Source: three-view drawing plus pictorial views. Frame: mm from the lowest corner of the part. A direction names the side the tool comes from. Round coordinates to 2 decimals unless told otherwise and drop trailing zeros. Loops run counter-clockwise (first coordinate to the right, second up) from the corner with the lowest first, then second, coordinate; pieces in that order, holes last. Notation, with made-up numbers: (3, -34.5) -> (26, -34.5) arc R15 cw to (26, -11.5) -> close; hole circle Ø8 at (38.25, 71.25). An arc over 180 degrees is marked (long way). Put each result on its own line as item: value. Start each with the question number.
1. Cut plane A-A (y = 45.5). Return the cut outline in (x, z).
2. Material intervals for L1, parallel to X at y = 60, z = 244.5; L2, parallel to Y at x = 130.5, z = 214; L3, parallel to Z at x = 33, y = 45.5, sorted ascending.
3. Contact query for flat-ended pins moving along their axis: pin 1 (23.5 mm diameter, centred on x = 72, y = 26.5, fed in from +Z); pin 2 (5 mm diameter, centred on y = 96, z = 177.5, fed in from -X); pin 3 (1.5 mm diameter, centred on x = 190.5, z = 207.5, fed in from -Y). Output: stop coordinate, or through.
4. Cut plane C-C (x = 24). Return the cut outline in (y, z).
5. Cut plane B-B (z = 37). Return the cut outline in (x, y).
6. Set-up query: the marked faces 1, 2 and 3. Return all of +Z, -Z, +X, -X, +Y, -Y with unobstructed straight access to the full face (end or side cutting, diameter ignored); none if empty.
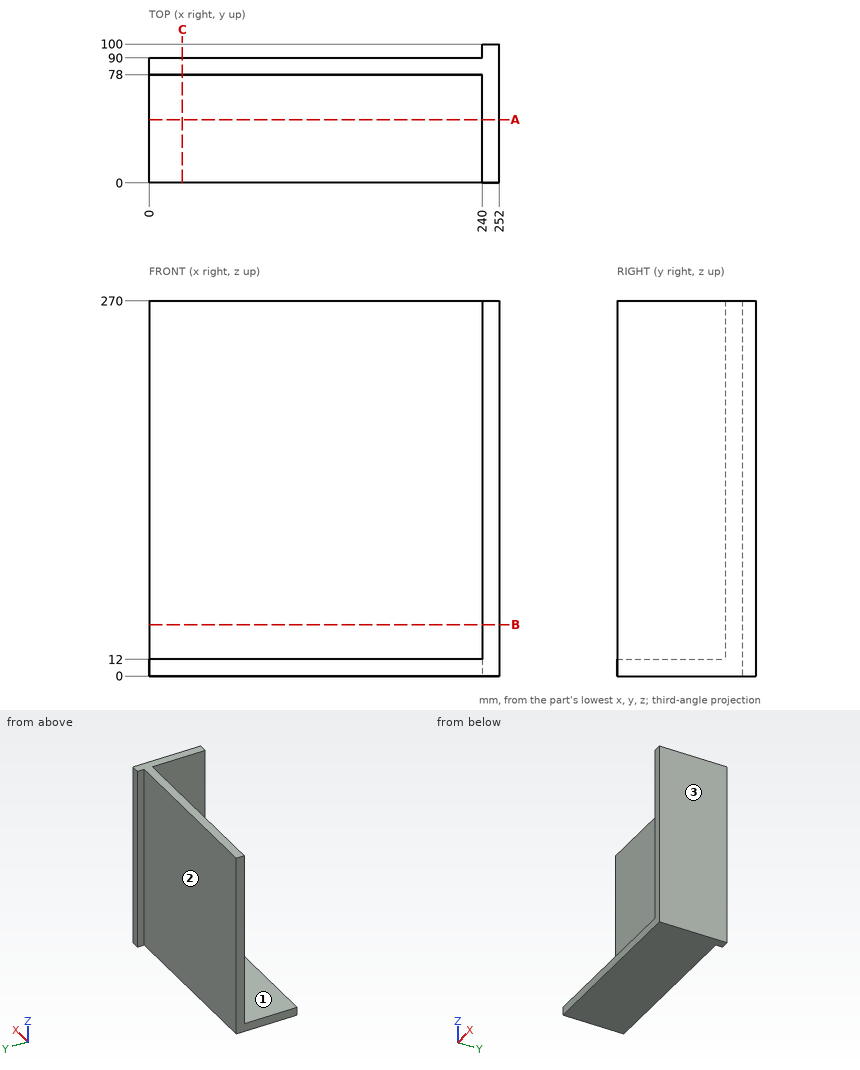
Solution:
1. outline: (0, 0) -> (252, 0) -> (252, 270) -> (240, 270) -> (240, 12) -> (0, 12) -> close
2. L1: x = 240 to 252
2. L2: y = 78 to 90
2. L3: z = 0 to 12
3. pin 1: stops at z = 12
3. pin 2: stops at x = 240
3. pin 3: stops at y = 78
4. outline: (0, 0) -> (90, 0) -> (90, 270) -> (78, 270) -> (78, 12) -> (0, 12) -> close
5. outline: (0, 78) -> (240, 78) -> (240, 0) -> (252, 0) -> (252, 100) -> (240, 100) -> (240, 90) -> (0, 90) -> close
6. face 1: +Z, -X, -Y
6. face 2: +Z, -Z, -X, +Y
6. face 3: +Z, -Z, +X, +Y, -Y
